Verification items for the finished model (mm, model axes). A direction names the side the tool comes from. Coordinates: 2 decimals unless noted, no trailing zeros. Loops run counter-clockwise (first coordinate to the right, second up) from the corner with the lowest first, then second, coordinate; pieces in that order, holes last. Notation, with made-up numbers: (10, 19.25) - (42, 19.25) arc R27 ccw to (42, 54.25) - close; hole circle Ø10 at (42.5, 11.25). An arc over 180 degrees is marked (long way). Answer as CSV lines item,"result". Start each with the question number.
1. Cross-section at B-B (z = -29.5). Enter the section's corners in (x, y), plus the area to 3 significant figures.
2. Set-up check for faces 1 (the flat face through (-98, 7.5, -19)), 2 (the flat face through (-103, 7.5, -19)), 3 (the cylindrical face through (-102.56, 4.96, -19.02)): record each of +Z, -Z, +X, -X, +Y, -Y from which the full face is reachable in a straight line by a thin tool's end or side.
3. Cross-section at A-A (y = 5.25). State how many separate pieces and enclosed holes the cut face has, plus the area to 3 significant figures.
4. Cross-section at C-C (x = -85). Enter the section's corners in (y, z).
5. Cross-section at D-D (z = -25.75). Enter the section's corners in (x, y), plus the area to 3 significant figures.
6. Material ranges on line 1 (X direction, y = 2.25, z = -19); line 2 (X direction, y = 5, z = -23.25); line 3 (X direction, y = 3, z = -29), recorded low to high. Write a range as [from, to].
7. Gauge pin test, flat ends, axial feed: P1, Ø1.5, axis at x = -74.5, y = 2, coming from the -Z side; P2, Ø2.5, axis at x = -76, y = 5, coming from the +Z side; P3, Ø0.8, axis at x = -58.5, z = -18.5, coming from the +Y side. Record the tip position at first contact, or that the pin passes through.
8. Release check for a two-part mould opening along X. For faces 4 (the flat face through (-54.6, 7.5, -19)), 5 (the cylindrical face through (-59.61, 4.96, -19.02)), 6 (the flat face through (-51.072, 0.5, -24.5)) record: pulls with the +X half, pulls with the -X half, needs draft (parallel to the pull), parting line crosses it, or undercut.
```python
from build123d import *

# Parameters (mm, degrees)
SKETCH1_W           = 56
SKETCH1_H           = 14
BOSS_EXTRUDE1_DEPTH = 1
SKETCH2_R           = 3.20517332
SKETCH2_R_2         = 4.024260076
SKETCH2_W           = 13.356664084
SKETCH2_H           = 12.745574878
BOSS_EXTRUDE2_DEPTH = 8
SKETCH3_W           = 10.103816096
SKETCH3_H           = 2.676767311
SKETCH3_W_2         = 10.213919594
BOSS_EXTRUDE4_DEPTH = 1.5
SKETCH4_R           = 0.58561586
SKETCH4_R_2         = 0.523790748
BOSS_EXTRUDE5_DEPTH = 5


with BuildPart() as part:
    # Sketch1 → Boss-Extrude1 (new body)
    with BuildSketch(Plane(origin=(0, 0, 0), x_dir=(1, 0, 0), z_dir=(0, 1, 0))):
        with Locations((-79.072208288, 24.556101007)):
            Rectangle(SKETCH1_W, SKETCH1_H)
    extrude(amount=BOSS_EXTRUDE1_DEPTH)

    # Sketch2 → Boss-Extrude2 (add)
    with BuildSketch(Plane(origin=(0, 1, 0), x_dir=(1, 0, 0), z_dir=(0, 1, 0))):
        with Locations(Location((-98.277869063, 25.472734817, 0), (0, 0, 270))):
            Circle(SKETCH2_R)
        with Locations(Location((-59.779249055, 26.520316314, 0), (0, 0, 270))):
            Circle(SKETCH2_R_2)
        with Locations((-72.917666994, 24.86164561)):
            Rectangle(SKETCH2_W, SKETCH2_H)
    extrude(amount=BOSS_EXTRUDE2_DEPTH)

    # Sketch3 → Boss-Extrude4 (add)
    with BuildSketch(Plane(origin=(0, 1, 0), x_dir=(1, 0, 0), z_dir=(0, 1, 0))):
        with Locations((-102.02030024, 18.894484663)):
            Rectangle(SKETCH3_W, SKETCH3_H)
        with Locations((-58.600719871, 18.894484663)):
            Rectangle(SKETCH3_W_2, SKETCH3_H)
    extrude(amount=BOSS_EXTRUDE4_DEPTH)

    # Sketch4 → Boss-Extrude5 (add)
    with BuildSketch(Plane(origin=(0, 2.5, 0), x_dir=(1, 0, 0), z_dir=(0, 1, 0))):
        with Locations(Location((-105.523641083, 18.948565176, 0), (0, 0, 270))):
            Circle(SKETCH4_R)
        with Locations(Location((-103.079284257, 18.948565176, 0), (0, 0, 270))):
            Circle(SKETCH4_R_2)
        with Locations(Location((-100.634927431, 18.948565176, 0), (0, 0, 270))):
            Circle(SKETCH4_R_2)
        with Locations(Location((-98.103272147, 18.948565176, 0), (0, 0, 270))):
            Circle(SKETCH4_R_2)
        with Locations(Location((-62.747396629, 18.948565176, 0), (0, 0, 270))):
            Circle(SKETCH4_R)
        with Locations(Location((-60.128442887, 18.948565176, 0), (0, 0, 270))):
            Circle(SKETCH4_R_2)
        with Locations(Location((-57.422190687, 18.948565176, 0), (0, 0, 270))):
            Circle(SKETCH4_R)
        with Locations(Location((-54.628640029, 18.948565176, 0), (0, 0, 270))):
            Circle(SKETCH4_R_2)
    extrude(amount=BOSS_EXTRUDE5_DEPTH)


solid = part.part
```
Values follow:
1,outline,"(-107.07, 0) - (-51.07, 0) - (-51.07, 1) - (-57.07, 1) - (-57.07, 9) - (-62.48, 9) - (-62.48, 1) - (-66.24, 1) - (-66.24, 9) - (-79.6, 9) - (-79.6, 1) - (-107.07, 1) - close"
1,area,"206 mm²"
2,face 1,"+Z, -X, +Y"
2,face 2,"+Z, -Z, -X, +Y"
2,face 3,"+Y"
3,separate pieces,"11"
3,enclosed holes,"0"
3,area,"261 mm²"
4,outline,"(0, -31.56) - (1, -31.56) - (1, -17.56) - (0, -17.56) - close"
5,outline,"(-107.07, 0) - (-51.07, 0) - (-51.07, 1) - (-55.83, 1) - (-55.83, 9) - (-63.73, 9) - (-63.73, 1) - (-66.24, 1) - (-66.24, 9) - (-79.6, 9) - (-79.6, 1) - (-95.08, 1) - (-95.08, 9) - (-101.47, 9) - (-101.47, 1) - (-107.07, 1) - close"
5,area,"277 mm²"
6,line 1,"x = [-107.07, -96.97], [-79.6, -66.24], [-63.71, -53.49]"
6,line 2,"x = [-100.59, -95.97], [-79.6, -66.24], [-62.12, -57.43]"
6,line 3,"x = [-79.6, -66.24], [-62.95, -56.61]"
7,P1,"stops at z = -31.23"
7,P2,"stops at z = -18.49"
7,P3,"stops at y = 2.5"
8,face 4,"needs draft"
8,face 5,"undercut"
8,face 6,"pulls with the +X half"
